Design review of the part built by this model. Coordinates are the model's own, in mm. Round coordinates to 2 decimals unless told otherwise and drop trailing zeros. Loops run counter-clockwise (first coordinate to the right, second up) from the corner with the lowest first, then second, coordinate; pieces in that order, holes last. Notation, with made-up numbers: (53, 86.5) - (102, 86.5) arc R16 ccw to (102, 95.5) - close; hole circle Ø4 at (17, -22). An arc over 180 degrees is marked (long way). Return JSON: item names as keys, results as strings. Group by question number.
(1) Wall thickness on L1, parallel to X at y = -7.75, z = 26.5; L2, parallel to Z at x = -84.5, y = -8.25; L3, parallel to X at y = -3, z = 19: over which ranges is each line inside the solid? List them lowest first. Write a range as [from, to].
(2) Clearance check with flat-ended pins moving along their axes: pin 1 (2 mm diameter, centred on y = -1, z = 11, fed in from -X); pin 2 (3 mm diameter, centred on y = -5, z = 8.5, fed in from +X); pin 3 (4 mm diameter, centred on y = -2.5, z = 20.5, fed in from +X). State where each tip first meets the part, or that it passes through.
(3) We need section A-A, the plane z = -29. Write out the cut boundary in (x, y).
(4) We need section B-B, the plane x = -1. Write out the cut boundary in (y, z).
(5) We need section C-C, the plane z = 19. Write out the cut boundary in (x, y).
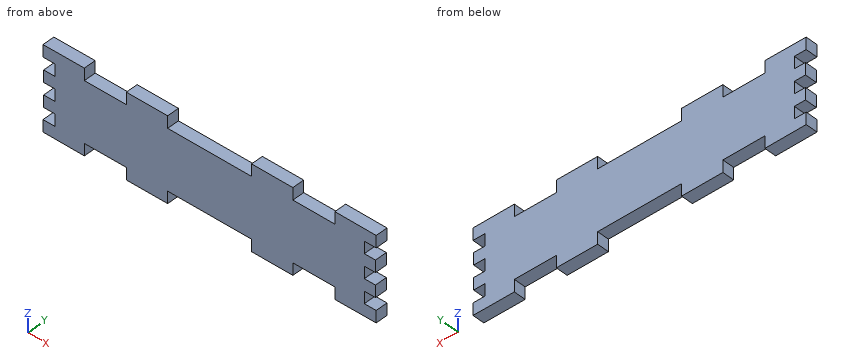
from build123d import *

# Parameters (mm, degrees)
F1_DEPTH = 10


with BuildPart() as f1:
    # F0 (on Front) → F1 (new body)
    with BuildSketch(Plane.XZ):
        Polygon((105.25, -35.124361), (140, -35), (140, -25), (130, -25), (130, -15), (139.429527, -15), (139.429527, -5), (130, -5), (130, 5), (139.429527, 5), (139.429527, 15), (130, 15), (130, 25), (140, 25), (140, 35), (105.25, 35.124361), (105.25, 25.124361), (70, 25.124361), (70, 35.124361), (35.25, 35.124361), (35.25, 25.124361), (0, 25.124361), (-35.25, 25.124361), (-35.25, 35.124361), (-70, 35.124361), (-70, 25.124361), (-105.25, 25.124361), (-105.25, 35.124361), (-140, 35), (-140, 25), (-130, 25), (-130, 15), (-139.429527, 15), (-139.429527, 5), (-130, 5), (-130, -5), (-139.429527, -5), (-139.429527, -15), (-130, -15), (-130, -25), (-140, -25), (-140, -35), (-105.25, -35.124361), (-105.25, -25.124361), (-70, -25.124361), (-70, -35.124361), (-35.25, -35.124361), (-35.25, -25.124361), (0, -25.124361), (35.25, -25.124361), (35.25, -35.124361), (70, -35.124361), (70, -25.124361), (105.25, -25.124361), align=None)
    extrude(amount=F1_DEPTH)


solid = f1.part
Solutions:
{
 "1": {"L1": "[-140, -105.25], [-70, -35.25], [35.25, 70], [105.25, 140]", "L2": "[-25.12, 25.12]", "L3": "[-130, 130]"},
 "2": {"pin 1": "x = -139.43", "pin 2": "x = 139.43", "pin 3": "x = 130"},
 "3": {"outline": "(-140, -10) - (-105.25, -10) - (-105.25, 0) - (-140, 0) - close; (-70, -10) - (-35.25, -10) - (-35.25, 0) - (-70, 0) - close; (35.25, -10) - (70, -10) - (70, 0) - (35.25, 0) - close; (105.25, -10) - (140, -10) - (140, 0) - (105.25, 0) - close"},
 "4": {"outline": "(-10, -25.12) - (0, -25.12) - (0, 25.12) - (-10, 25.12) - close"},
 "5": {"outline": "(-130, -10) - (130, -10) - (130, 0) - (-130, 0) - close"}
}
